Here's how the part is built. I have some questions about the finished solid (model axes, mm). Face numbers are marked on the shaded views. A direction names the side the tool comes from. Give positions to 0.01 mm unless a question says otherwise; leave off trailing zeros. Loops run counter-clockwise (first coordinate to the right, second up) from the corner with the lowest first, then second, coordinate; pieces in that order, holes last. Notation, with made-up numbers: (-38, 39.25) - (8, 39.25) arc R24 ccw to (8, 58.25) - close; hole circle Ø5 at (-7, 64.5). An arc over 180 degrees is marked (long way). Use one line per item in the form item = value.
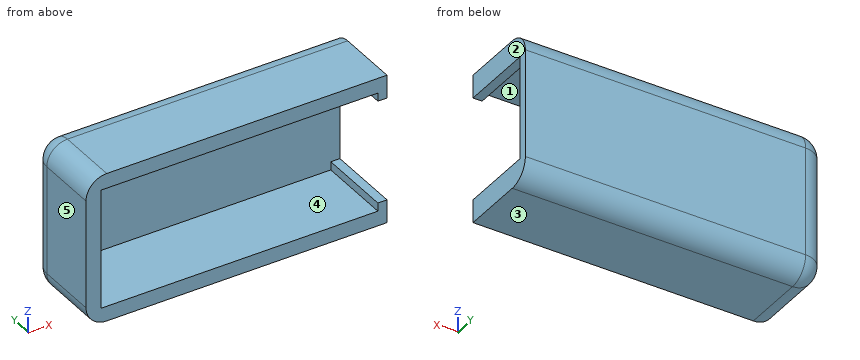
from build123d import *

# Parameters (mm, degrees)
SKETCH_1_W          = 72.2
SKETCH_1_H          = 36.2
SKETCH_1_W_2        = 65
SKETCH_1_H_2        = 29
EXTRUDE_1_DEPTH     = 20
SKETCH_2_W          = 29
SKETCH_2_H          = 20
CUT_EXTRUDE_1_DEPTH = 3.6
SKETCH_3_W          = 3.6
SKETCH_3_H          = 20
EXTRUDE_1_2_DEPTH   = 0.6
SKETCH_4_W          = 2.2
SKETCH_4_H          = 20
EXTRUDE_2_DEPTH     = 2
SKETCH_5_W          = 2.2
SKETCH_5_H          = 20
EXTRUDE_3_DEPTH     = 2
SKETCH_6_W          = 72.8
SKETCH_6_H          = 36.2
EXTRUDE_4_DEPTH     = 2
FILLET_1_R          = 5
FILLET_2_R          = 5
FILLET_3_R          = 5


with BuildPart() as part:
    # 草图1 → Extrude 1 (new body)
    with BuildSketch(Plane(origin=(0, 0, 0), x_dir=(1, 0, 0), z_dir=(0, 1, 0))):
        with Locations((32.5, 14.5)):
            Rectangle(SKETCH_1_W, SKETCH_1_H)
        with Locations((32.5, 14.5)):
            Rectangle(SKETCH_1_W_2, SKETCH_1_H_2, mode=Mode.SUBTRACT)
    extrude(amount=EXTRUDE_1_DEPTH)

    # 草图2 → 切除-拉伸1 (cut)
    with BuildSketch(Plane.ZY.offset(-65)):
        with Locations((-14.5, 10)):
            Rectangle(SKETCH_2_W, SKETCH_2_H)
    extrude(amount=-CUT_EXTRUDE_1_DEPTH, mode=Mode.SUBTRACT)

    # 草图3 → Extrude 1 2 (add)
    with BuildSketch(Plane(origin=(68.6, 0, 0), x_dir=(0, 0, -1), z_dir=(1, 0, 0))):
        with Locations((-1.8, 10)):
            Rectangle(SKETCH_3_W, SKETCH_3_H)
        with Locations((30.8, 10)):
            Rectangle(SKETCH_3_W, SKETCH_3_H)
    extrude(amount=EXTRUDE_1_2_DEPTH)

    # 草图4 → 凸台-拉伸2 (add)
    with BuildSketch(Plane(origin=(0, 0, 0), x_dir=(-1, 0, 0), z_dir=(0, 0, -1))):
        with Locations((-68.1, 10)):
            Rectangle(SKETCH_4_W, SKETCH_4_H)
    extrude(amount=EXTRUDE_2_DEPTH)

    # 草图5 → 凸台-拉伸3 (add)
    with BuildSketch(Plane.XY.offset(-29)):
        with Locations((68.1, 10)):
            Rectangle(SKETCH_5_W, SKETCH_5_H)
    extrude(amount=EXTRUDE_3_DEPTH)

    # 草图6 → 凸台-拉伸4 (add)
    with BuildSketch(Plane(origin=(0, 20, 0), x_dir=(1, 0, 0), z_dir=(0, 1, 0))):
        with Locations((32.8, 14.5)):
            Rectangle(SKETCH_6_W, SKETCH_6_H)
    extrude(amount=-EXTRUDE_4_DEPTH)

    # 圆角1
    fillet_1_edges = [part.edges().sort_by_distance(p)[0] for p in [
        (32.8, 20, -32.6),
    ]]
    fillet(fillet_1_edges, radius=FILLET_1_R)

    # 圆角2
    fillet_2_edges = [part.edges().sort_by_distance(p)[0] for p in [
        (32.8, 20, 3.6),
    ]]
    fillet(fillet_2_edges, radius=FILLET_2_R)

    # 圆角3
    fillet_3_edges = [part.edges().sort_by_distance(p)[0] for p in [
        (-3.6, 20, -14.5),
        (-3.6, 7.5, -32.6),
        (-3.6, 18.535533906, -31.135533906),
        (-3.6, 7.5, 3.6),
        (-3.6, 18.535533906, 2.135533906),
    ]]
    fillet(fillet_3_edges, radius=FILLET_3_R)


solid = part.part
(1) If we section it at B-B (z = -23): List the corners of the cut face in (x, y) for me, plus the area to 3 significant figures.
Geometry says:
outline = (-3.6, 0) - (0, 0) - (0, 18) - (69.2, 18) - (69.2, 20) - (1.4, 20) arc R5 ccw to (-3.6, 15) - close
area = 205 mm²
(2) If we section it at C-C (x = 63): List the corners of the cut face in (y, z) for me, plus the area to 3 significant figures.
Geometry says:
outline = (0, -32.6) - (15, -32.6) arc R5 ccw to (20, -27.6) - (20, -1.4) arc R5 ccw to (15, 3.6) - (0, 3.6) - (0, 0) - (18, 0) - (18, -29) - (0, -29) - close
area = 191 mm²
(3) If we section it at A-A (y = 9): List the corners of the cut face in (x, z) for me, plus the area to 3 significant figures.
Geometry says:
outline = (-3.6, -27.6) arc R5 ccw to (1.4, -32.6) - (69.2, -32.6) - (69.2, -27) - (67, -27) - (67, -29) - (0, -29) - (0, 0) - (67, 0) - (67, -2) - (69.2, -2) - (69.2, 3.6) - (1.4, 3.6) arc R5 ccw to (-3.6, -1.4) - close
area = 627 mm²
(4) If I drill on probe 1 along Z at (x, y) = (35.5, 6.25); probe 2 along X at (y, z) = (2.75, -28); probe 3 along Y at (x, z) = (28.5, -12), over which ranges is the centre line in solid material (lowest first)?
Geometry says:
probe_1 = -32.6 to -29, 0 to 3.6
probe_2 = -3.58 to 0, 67 to 69.2
probe_3 = 18 to 20
(5) Thinking about a two-plate mould opening in X: for the marked faces 1, 2 and 3, which applies, pulls with the +X half, pulls with the -X half, needs draft (parallel to the pull), parting line crosses it, or undercut?
Geometry says:
face_1 = undercut
face_2 = pulls with the +X half
face_3 = needs draft
(6) For P1, Ø1, axis at y = 14.5, z = -0.5, coming from the -X side; P2, Ø5, axis at x = 31.5, z = -22.5, coming from the -Y side; P3, Ø5.5, axis at y = 5, z = -9.5, coming from the +X side, each with a flat end and sliding along its axis, tell me the tip position at first contact or that it passes through.
Geometry says:
P1 = -3.58
P2 = 18
P3 = 0
(7) For the marked faces 4 and 5, which set-ups out of +Z, -Z, +X, -X, +Y, -Y let a thin tool reach every point of the face, with its end or its side?
Geometry says:
face_4 = -Y
face_5 = +Z, -Z, -X, +Y, -Y
